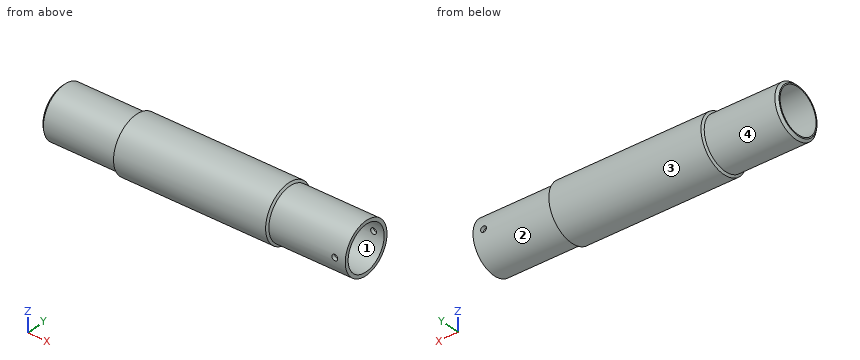
Autodesk Inventor part; units mm, degrees
ref_plane "YZ Plane" through (0, 0, 0) normal (1, 0, 0) x (0, 1, 0)
ref_plane "XZ Plane" through (0, 0, 0) normal (0, 1, 0) x (-1, 0, 0)
ref_plane "XY Plane" through (0, 0, 0) normal (0, 0, 1) x (1, 0, 0)
sketch "Profile" plane through (0, 0, 0) normal (0, 0, 1) x (1, 0, 0)
  line L0 (-31.2, 0) -> (-31.2, 11)
  line L1 (-31.2, 11) -> (0, 11)
  line L2 (0, 11) -> (0.5774, 12)
  line L3 (0.5774, 12) -> (65.5774, 12)
  line L4 (65.5774, 12) -> (66.1547, 11)
  line L5 (66.1547, 11) -> (98.8, 11)
  line L6 (98.8, 11) -> (98.8, 0)
  line L7 (-31.2, 0) -> (0, 0)
  line L8 (0, 0) -> (0, 9)
  line L9 (0, 9) -> (90.8, 9)
  line L10 (90.8, 9) -> (90.8, 0)
  line L11 (90.8, 0) -> (98.8, 0)
  line L12 (-57.2, 0) -> (124.8, 0) construction
  line L13 (0, 11) -> (0, 9) construction
  dimension "BodyLength" = 130
  dimension "d1" = 11
  dimension "d3" = 120
  dimension "d4" = 120
  dimension "d5" = 65
  dimension "d6" = 31.2
  dimension "d16" = 8
  dimension "d29" = 1
  dimension "d30" = 9
revolve "ProfileRevolveFeature" add sketch "Profile" angle 360 about axis through (-10, 0, 0) along (1, 0, 0)
sketch "InsideHole" plane through (-31.2, 0, 0) normal (-1, 0, 0) x (0, 0, 1)
  circle A0 centre (0, 0) radius 9 construction
hole "InsideHoleFeature" at (-31.2, 0, 0) direction (1, 0, 0) diameter 19 end through all
chamfer "EndChamferFeature" distance 1 angle 45 1 edges at (-31.2, -11, 0)
sketch "CapMountHole" plane through (0, 0, 0) normal (0, 1, 0) x (-1, 0, 0)
  line L0 (-98.8, 11) -> (-98.8, -11) construction
  line L1 (5.32, 0) -> (-31.92, 0) construction
  circle A0 centre (-94.3, 0) radius 1.25
  point P0 (0, 0)
  dimension "d31" = 4.5
  dimension "d39" = 2.5
extrude "CapMountHoleFeature" cut sketch "CapMountHole" along normal through all both and the other way through all
equation "\"d5\" = 0.5 * BodyLength"
equation "\"d6\" = 0.24 * BodyLength"
properties part number "BackPair1PistonBody"
Read the model definition and answer for the solid it produces. Units are mm, in the model's axes. Face numbers are marked on the shaded views. A direction names the side the tool comes from. Coordinates: 2 decimals unless noted, no trailing zeros. Write each loop counter-clockwise with the first axis right and the second up, starting at its lowest first coordinate (ties: lowest second). Pieces come first, ordered by that corner, then holes. Notation, with made-up numbers: (59, -2) -> (112, -2) arc R28 cw to (112, 24) -> close; hole circle Ø1 at (19, 74.25). An arc over 180 degrees is marked (long way). Return JSON: item names as keys, results as strings.
(1) The part is cut by section D-D on x = 18. Give the vertices of the cut face in (y, z), then the cut area to 3 significant figures.
Answers below:
{"outline": "circle Ø24 at (0, 0); hole circle Ø19 at (0, 0)", "area": "169 mm^2"}
(2) For a pull along Y with two mould halves and no side action, classify the marked faces 1 and 2 as pulls with the +Y half, pulls with the -Y half, needs draft (parallel to the pull), parting line crosses it, or undercut.
Answers below:
{"face 1": "undercut", "face 2": "parting line crosses it"}
(3) The part is cut by section A-A on y = 0. Give the vertices of the cut face in (x, z).
Answers below:
{"outline": "(-31.2, -10) -> (-30.2, -11) -> (0, -11) -> (0.58, -12) -> (65.58, -12) -> (66.15, -11) -> (98.8, -11) -> (98.8, -9.5) -> (-31.2, -9.5) -> close; (-31.2, 9.5) -> (98.8, 9.5) -> (98.8, 11) -> (66.15, 11) -> (65.58, 12) -> (0.58, 12) -> (0, 11) -> (-30.2, 11) -> (-31.2, 10) -> close"}
(4) Which of the six approach directions +Z, -Z, +X, -X, +Y, -Y give full straight-line access (tool end or side, diameter ignored) to the marked faces 3 and 4?
Answers below:
{"face 3": "+X, -X", "face 4": "-X"}
(5) Consider line 1 along Z through (x, y) = (24, 0); line 2 along X through (y, z) = (10.5, 0); line 3 along Z through (x, y) = (-21, 2.25). Determine where each line is inside the solid, lowest interval first. Write a range as from..to.
Answers below:
{"line 1": "-12..-9.5, 9.5..12", "line 2": "-30.7..93.05, 95.55..98.8", "line 3": "-10.77..-9.23, 9.23..10.77"}
(6) The part is cut by section B-B on z = 0. Give the vertices of the cut face in (x, y), then the cut area to 3 significant figures.
Answers below:
{"outline": "(-31.2, -10) -> (-30.2, -11) -> (0, -11) -> (0.58, -12) -> (65.58, -12) -> (66.15, -11) -> (93.05, -11) -> (93.05, -9.5) -> (-31.2, -9.5) -> close; (-31.2, 9.5) -> (93.05, 9.5) -> (93.05, 11) -> (66.15, 11) -> (65.58, 12) -> (0.58, 12) -> (0, 11) -> (-30.2, 11) -> (-31.2, 10) -> close; (95.55, -11) -> (98.8, -11) -> (98.8, -9.5) -> (95.55, -9.5) -> close; (95.55, 9.5) -> (98.8, 9.5) -> (98.8, 11) -> (95.55, 11) -> close", "area": "513 mm^2"}
(7) Each of these flat-tipped pins is pushed along its axis until it touches: P1, Ø2, axis at y = 9, z = 2.5, coming from the +X side; P2, Ø1.5, axis at x = 27, y = -7.5, coming from the -Z side; P3, Ø8, axis at y = -2, z = -0.5, coming from the -X side; P4, Ø1, axis at x = 45.5, y = -6, coming from the +Z side. Where does it stop, or does it pass through?
Answers below:
{"P1": "x = 98.8", "P2": "z = -9.92", "P3": "through", "P4": "z = 10.67"}
(8) The part is cut by section C-C on x = 94.3. Give the vertices of the cut face in (y, z), then the cut area to 3 significant figures.
Answers below:
{"outline": "(-10.93, -1.25) arc R11 ccw to (10.93, -1.25) -> (9.42, -1.25) arc R9.5 cw to (-9.42, -1.25) -> close; (-10.93, 1.25) -> (-9.42, 1.25) arc R9.5 cw to (9.42, 1.25) -> (10.93, 1.25) arc R11 ccw to start", "area": "89.1 mm^2"}
